Part model, mm, in its own coordinate system. Face numbers are marked on the shaded views. A direction names the side the tool comes from. Give positions to 0.01 mm unless a question says otherwise; leave off trailing zeros. Loops run counter-clockwise (first coordinate to the right, second up) from the corner with the lowest first, then second, coordinate; pieces in that order, holes last. Notation, with made-up numbers: M 8,72 L 63,72 A5 ccw 63,81 Z; hole C 34,-1.75 d10. An arc over 180 degrees is marked long. Put each result on its own line as item: value. Start each with the question number.
Autodesk Inventor part; units mm, degrees
ref_plane "YZ Plane" through (0, 0, 0) normal (1, 0, 0) x (0, 1, 0)
ref_plane "XZ Plane" through (0, 0, 0) normal (0, 1, 0) x (-1, 0, 0)
ref_plane "XY Plane" through (0, 0, 0) normal (0, 0, 1) x (1, 0, 0)
sketch "Sketch1" plane through (0, 0, 0) normal (0, 1, 0) x (-1, 0, 0)
  line L0 (6, -3.5) -> (-6, -3.5)
  line L1 (-6, -3.5) -> (-6, 3.5)
  line L2 (-6, 3.5) -> (6, 3.5)
  line L3 (6, 3.5) -> (6, -3.5)
  line L4 (6, -3.5) -> (-6, 3.5) construction
  line L5 (-6, -3.5) -> (6, 3.5) construction
  point P0 (0, 0)
  dimension "d0" = 12
  dimension "d1" = 7
extrude "Extrusion1" add sketch "Sketch1" along normal blind 9
sketch "Sketch2" plane through (0, 9, 0) normal (0, 1, 0) x (1, 0, 0)
  circle A0 centre (0, 0) radius 3
  dimension "d4" = 6
extrude "Extrusion2" add sketch "Sketch2" along normal blind 9
sketch "Sketch5" plane through (0, 0, 0) normal (0, 0, 1) x (1, 0, 0)
  line L0 (3, 18) -> (-3, 18) construction
  line L1 (-3, 9) -> (3, 9) construction
  line L2 (0, 18) -> (0, 28)
  line L3 (0, 18) -> (1, 18)
  line L4 (1, 18) -> (1.7768, 26.8789)
  arc A0 (0.8673, 27.9623) -> (0, 28) centre (0, 18) ccw
  arc A1 (0, 28) -> (1.8596, 27.8256) centre (0, 18) ccw construction
  arc A2 (1.7768, 26.8789) -> (0.8673, 27.9623) centre (0.7806, 26.9661) ccw
  point P0 (0, 0)
  dimension "d7" = 10
  dimension "d8" = 1
  dimension "d9" = 85
  dimension "d10" = 1
revolve "Revolution1" add sketch "Sketch5" angle 360 about axis through (0, 18, 0) along (0, 1, 0)
thread "Thread1"
properties part number "Switch"
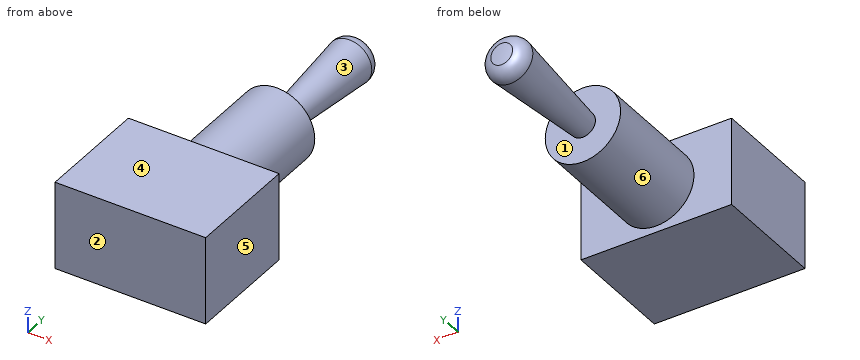
1) Pin check, flat tips, straight feed: pin 1 Ø4 at (x, z) = (-4, -1) entering from +Y; pin 2 Ø2 at (x, z) = (2, -1.5) entering from +Y; pin 3 Ø4 at (y, z) = (18.5, -2) entering from -X; pin 4 Ø1 at (x, z) = (3, -2.5) entering from -Y. Stop position of each tip, or through.
2) Band-saw the part on A-A on y = 22.5. Give the cut face in (x, z), then the cut area to 3 significant figures.
3) Mould opens along Y. For the marked faces 1, 2, 3 and 4 say: +Y half, -Y half, draft (parallel to the pull), parting line (faces both ways), or undercut.
4) Which spindle directions (+Z, -Z, +X, -X, +Y, -Y) get a long thin tool onto all of the face, cutting with end or side? Do the marked faces 5 and 6. Say none if no direction does.
5) Wall check: L1, parallel to Y at x = 3.5, z = 2; L2, parallel to X at y = 12.25, z = 0; L3, parallel to Y at x = 0.5, z = -2.5. Give the ranges that are in metal, low to high.
Evaluation:
1. pin 1: y = 18
1. pin 2: y = 27.66
1. pin 3: x = -3
1. pin 4: y = 0
2. outline: C 0,0 d2.79
2. area: 6.10 mm2
3. face 1: undercut
3. face 2: -Y half
3. face 3: undercut
3. face 4: draft
4. face 5: +Z, -Z, +X, +Y, -Y
4. face 6: +Y
5. L1: 0 to 9
5. L2: -3 to 3
5. L3: 0 to 18
